```python
from build123d import *

# Parameters (mm, degrees)
F0_R     = 6.3246
F0_R_2   = 4.7879
F1_DEPTH = 20.32
F2_DEPTH = 4.572
F3_SIZE  = 1.016


with BuildPart() as f1:
    # F0 (on Front) → F1 (new body)
    with BuildSketch(Plane.XZ):
        Circle(F0_R)
        Circle(F0_R_2, mode=Mode.SUBTRACT)
    extrude(amount=F1_DEPTH)

    # F0 (on Front) → F2 (join)
    with BuildSketch(Plane.XZ):
        Polygon((7.015579, -5.898039), (8.615641, 3.12665), (1.600062, 9.024689), (-7.015579, 5.898039), (-8.615641, -3.12665), (-1.600062, -9.024689), align=None)
        Circle(F0_R, mode=Mode.SUBTRACT)
    extrude(amount=F2_DEPTH)

    # F3
    f3_edges = [f1.edges().sort_by_distance(p)[0] for p in [
        (-4.7879, -20.32, 0),
    ]]
    chamfer(f3_edges, length=F3_SIZE)


solid = f1.part
```
Input: part model. Units: mm. Frame: model coordinates. A direction names the side the tool comes from. Give positions to 0.01 mm unless a question says otherwise; leave off trailing zeros. Order: outer loops, then holes, each group sorted by start corner. A loop starts at its lowest first (then second) coordinate and runs counter-clockwise, first axis right, second up. Notation, with made-up numbers: (17.25, 65.5) - (54.25, 65.5) arc R17 cw to (54.25, 72.5) - close; hole circle Ø2 at (-38, 45). An arc over 180 degrees is marked (long way). Put each result on its own line as item: value.
Item 1: Section query D-D, the plane y = -10.5. Return loops of the section in (x, z), then the cut area to 3 significant figures.
Found:
outline: circle Ø12.65 at (0, 0); hole circle Ø9.58 at (0, 0)
area: 53.6 mm^2
Item 2: Section query A-A, the plane y = -3.25. Return loops of the section in (x, z).
Found:
outline: (-8.62, -3.13) - (-1.6, -9.02) - (7.02, -5.9) - (8.62, 3.13) - (1.6, 9.02) - (-7.02, 5.9) - close; hole circle Ø9.58 at (0, 0)
Item 3: Contact query for flat-ended pins moving along their axis: pin 1 (4 mm diameter, centred on y = -9, z = -1, fed in from +X); pin 2 (1 mm diameter, centred on x = 1.5, y = -9.5, fed in from -Z); pin 3 (7.5 mm diameter, centred on x = 0, z = 0, fed in from -Y); pin 4 (1 mm diameter, centred on x = -6, y = -2, fed in from -Z). Output: stop coordinate, or through.
Found:
pin 1: stops at x = 6.32
pin 2: stops at z = -6.25
pin 3: passes through
pin 4: stops at z = -5.75
Item 4: Section query C-C, the plane z = 0. Return loops of the section in (x, y).
Found:
outline: (-8.06, -4.57) - (-6.32, -4.57) - (-6.32, -20.32) - (-5.8, -20.32) - (-4.79, -19.3) - (-4.79, 0) - (-8.06, 0) - close; (4.79, -19.3) - (5.8, -20.32) - (6.32, -20.32) - (6.32, -4.57) - (8.06, -4.57) - (8.06, 0) - (4.79, 0) - close
Item 5: Draft query along Z for faces 1 (the cylindrical face through (4.567, -9.517, 1.438)), 2 (the flat face through (7.804, -2.254, -1.449)), 3 (the flat face through (-7.804, -2.254, 1.449)). Return one class per face: +Z half, -Z half, draft (parallel to the pull), parting line (faces both ways), or undercut.
Found:
face 1: undercut
face 2: -Z half
face 3: +Z half
Item 6: Access query for faces 4 (the cylindrical face through (6, -12, 2)), 5 (the flat face through (5.2, -2.3, 6)). Directions: +Z, -Z, +X, -X, +Y, -Y. A direction counts if a zero-diameter tool reaches every point of the face in a straight line with its end or side. Return the directions, or none.
Found:
face 4: -Y
face 5: +Z, +X, +Y, -Y
Item 7: Ray query, L1, parallel to Z at x = 0, y = -10; L2, parallel to Y at x = 4.75, z = 6.25; L3, parallel to X at y = -11, z = -2.5. Return the intervals inside material, ascending. Write a range as from..to.
Found:
L1: z = -6.32..-4.79, 4.79..6.32
L2: y = -4.57..0
L3: x = -5.81..-4.08, 4.08..5.81
Item 8: Section query B-B, the plane x = 0. Return loops of the section in (y, z).
Found:
outline: (-20.32, -6.32) - (-4.57, -6.32) - (-4.57, -8.44) - (0, -8.44) - (0, -4.79) - (-19.3, -4.79) - (-20.32, -5.8) - close; (-20.32, 5.8) - (-19.3, 4.79) - (0, 4.79) - (0, 8.44) - (-4.57, 8.44) - (-4.57, 6.32) - (-20.32, 6.32) - close
